Check sheet for the modelled part. Datum: model origin and axes. Units: mm. Face numbers are marked on the shaded views. A direction names the side the tool comes from. Coordinates: 2 decimals unless noted, no trailing zeros. Loops run counter-clockwise (first coordinate to the right, second up) from the corner with the lowest first, then second, coordinate; pieces in that order, holes last. Notation, with made-up numbers: M 77,54.5 L 91,54.5 A9 cw 91,64.5 Z; hole C 78,83.25 d9. An arc over 180 degrees is marked long. Answer as CSV lines item,"result". Start each with the question number.
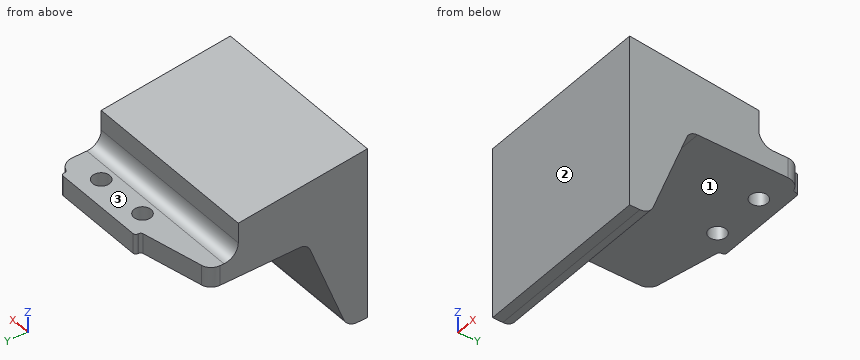
Autodesk Inventor part; units mm, degrees
ref_plane "YZ Plane" through (0, 0, 0) normal (1, 0, 0) x (0, 1, 0)
ref_plane "XZ Plane" through (0, 0, 0) normal (0, 1, 0) x (-1, 0, 0)
ref_plane "XY Plane" through (0, 0, 0) normal (0, 0, 1) x (1, 0, 0)
sketch "Sketch2" plane through (0, 0, 0) normal (1, 0, 0) x (0, 1, 0)
  line L0 (0, 0) -> (0, -30.48)
  line L1 (0, -30.48) -> (3.556, -30.48)
  line L2 (3.556, -30.48) -> (10.6288, -12.0547)
  line L3 (10.6288, -12.0547) -> (30.48, -12.0547)
  line L4 (30.48, -12.0547) -> (30.48, -8.4987)
  line L5 (30.48, -8.4987) -> (22.86, -8.4987)
  line L6 (22.86, -8.4987) -> (22.86, -2.4027)
  line L7 (22.86, -2.4027) -> (0, 0)
  dimension "d0" = 30.48
  dimension "d1" = 21
  dimension "d2" = 84
  dimension "d3" = 30.48
  dimension "d4" = 22.86
  dimension "d5" = 3.556
  dimension "d6" = 9.652
  dimension "d7" = 3.556
extrude "Extrusion1" add sketch "Sketch2" along normal mid plane 32.004
sketch "Sketch3" plane through (-16.002, 22.86, -8.4987) normal (0, 0, 1) x (1, 0, 0)
  line L0 (0, 7.62) -> (0, -12.2312)
  line L1 (0, 7.62) -> (12.7, 7.62)
  line L2 (0, 7.62) -> (32.004, 7.62)
  line L3 (0, 4.9205) -> (0, 7.62)
  line L4 (0, 4.9205) -> (12.7, 7.62)
  point P0 (16.002, -22.86)
  dimension "d10" = 12
  dimension "d11" = 12.7
extrude "Extrusion2" cut sketch "Sketch3" against normal blind 32.004
sketch "Sketch4" plane through (-16.002, 22.86, -8.4987) normal (0, 0, 1) x (1, 0, 0)
  line L0 (0, 4.9205) -> (12.7, 7.62)
  line L1 (12.7, 7.62) -> (29.972, 7.62)
  line L2 (29.972, 7.62) -> (29.972, 8.636)
  line L3 (29.972, 8.636) -> (12.7, 8.636)
  line L4 (12.7, 8.636) -> (12.7, 7.62)
  line L5 (32.004, 7.62) -> (32.004, 0)
  point P0 (16.002, -22.86)
  dimension "d15" = 1.016
  dimension "d18" = 17.272
extrude "Extrusion3" add sketch "Sketch4" against normal up to surface (3.556 mm away)
fillet "Fillet1" radius 2.54 1 edges at (0, 22.86, -8.4987)
fillet "Fillet2" radius 2.032 1 edges at (-16.002, 27.7805, -10.2767)
fillet "Fillet3" radius 2.54 1 edges at (16.002, 30.48, -10.2767)
fillet "Fillet4" radius 2.032 1 edges at (0, 10.6288, -12.0547)
fillet "Fillet4" radius 2.54 1 edges at (0, 3.556, -30.48)
fillet "Fillet4" radius 0.508 4 edges at (13.97, 30.48, -10.2767) (13.97, 31.496, -10.2767) (-3.302, 31.496, -10.2767) (-3.302, 30.48, -10.2767)
sketch "Sketch5" plane through (-16.002, 22.86, -8.4987) normal (0, 0, 1) x (1, 0, 0)
  line L0 (0, 0) -> (32.004, 0)
  line L1 (32.004, 7.62) -> (32.004, 0)
  point P0 (16.002, -22.86)
  point P1 (16.002, 4.826)
  point P2 (25.654, 4.826)
  dimension "d28" = 9.652
  dimension "d29" = 4.826
  dimension "d30" = 6.35
hole "Hole2" at (0, 27.686, -8.4987) at (9.652, 27.686, -8.4987) direction (0, 0, -1) diameter 3.048 end through all
Item 1: Sectioned sample at A-A, the plane x = 0. Record the boundary of the cut face in (y, z).
Item 2: Sectioned sample at B-B, the plane z = -5.5. Record the boundary of the cut face in (x, y).
Item 3: Set-up check for the marked faces 1, 2 and 3: record each of +Z, -Z, +X, -X, +Y, -Y from which the full face is reachable in a straight line by a thin tool's end or side.
Item 4: Sectioned sample at D-D, the plane x = -7.5. Record the boundary of the cut face in (y, z), and give its area (3 significant figures).
Item 5: Go/stop test with flat-tipped pins: pin 1 (5 mm diameter, centred on x = 1.5, y = 5, fed in from +Z); pin 2 (6 mm diameter, centred on x = -11, y = 5, fed in from +Z); pin 3 (1.5 mm diameter, centred on y = 24, z = -14.5, fed in from +X); pin 4 (1.5 mm diameter, centred on x = 5.5, z = -21.5, fed in from +Y). Record where each tip stops, or that it passes through.
Item 6: Material ranges on line 1 (Y direction, x = 0, z = -10); line 2 (Z direction, x = -2, y = 27); line 3 (Y direction, x = 13.5, z = -10), recorded low to high. Write a range as from..to.
Item 7: Sectioned sample at C-C, the plane y = 14.5. Record the boundary of the cut face in (x, z), and give its area (3 significant figures).
Reply:
1,outline,"M 0,-30.48 L 1.81,-30.48 A2.54 ccw 4.18,-28.85 L 10.13,-13.36 A2.03 cw 12.03,-12.05 L 26.16,-12.05 L 26.16,-8.5 L 25.4,-8.5 A2.54 cw 22.86,-5.96 L 22.86,-2.4 L 0,0 Z; M 29.21,-12.05 L 31.5,-12.05 L 31.5,-8.5 L 29.21,-8.5 Z"
2,outline,"M -16,0 L 16,0 L 16,22.86 L -16,22.86 Z"
3,face 1,"-Z, +X, -X, +Y"
3,face 2,"+Z, -Z, +X, -X, -Y"
3,face 3,"+Z, +X, -X, +Y"
4,outline,"M 0,-30.48 L 1.81,-30.48 A2.54 ccw 4.18,-28.85 L 10.13,-13.36 A2.03 cw 12.03,-12.05 L 29.59,-12.05 L 29.59,-8.5 L 25.4,-8.5 A2.54 cw 22.86,-5.96 L 22.86,-2.4 L 0,0 Z"
4,area,"404 mm²"
5,pin 1,"z = -0.26"
5,pin 2,"z = -0.21"
5,pin 3,"through"
5,pin 4,"y = 7.29"
6,line 1,"0..26.16, 29.21..31.5"
6,line 2,"-12.05..-8.5"
6,line 3,"0..31.49"
7,outline,"M -16,-12.05 L 16,-12.05 L 16,-1.52 L -16,-1.52 Z"
7,area,"337 mm²"
